from build123d import *

# Parameters (mm, degrees)
SKETCH1_W           = 76
SKETCH1_H           = 13
SKETCH1_W_2         = 74.5
SKETCH1_H_2         = 11.5
BOSS_EXTRUDE1_DEPTH = 2.5
SKETCH2_R           = 1.6
CUT_EXTRUDE1_DEPTH  = 41.239905566
BOSS_EXTRUDE2_REACH = 42.004
SKETCH3_R           = 1


with BuildPart() as part:
    # Sketch1 → Boss-Extrude1 (new, symmetric)
    with BuildSketch(Plane(origin=(0, 0, 0), x_dir=(1, 0, 0), z_dir=(0, 1, 0))):
        Rectangle(SKETCH1_W, SKETCH1_H)
        Rectangle(SKETCH1_W_2, SKETCH1_H_2, mode=Mode.SUBTRACT)
    extrude(amount=BOSS_EXTRUDE1_DEPTH, both=True)

    # Sketch2 → Cut-Extrude1 (cut, through all)
    with BuildSketch(Plane.XY.offset(6.5)):
        with Locations((23, 0)):
            Circle(SKETCH2_R)
        with BuildLine():
            Line((-25, 1.15), (8.6, 1.15))
            ThreePointArc((8.6, 1.15), (9.75, 0), (8.6, -1.15))
            Line((8.6, -1.15), (-25, -1.15))
            ThreePointArc((-25, -1.15), (-26.15, 0), (-25, 1.15))
        make_face()
    extrude(amount=-CUT_EXTRUDE1_DEPTH, mode=Mode.SUBTRACT)

    # Sketch3 → Boss-Extrude2 (add, up to next)
    with BuildSketch(Plane.XY.offset(-5.75), mode=Mode.PRIVATE) as boss_extrude2_sk1:
        with Locations(Location((-31, 0, 0), (0, 0, 180))):
            Circle(SKETCH3_R)
    boss_extrude2_tool1 = extrude(boss_extrude2_sk1.sketch, amount=BOSS_EXTRUDE2_REACH, mode=Mode.PRIVATE) - part.part
    add(boss_extrude2_tool1.solids().sort_by_distance((-31, 0, -5.75))[0])


solid = part.part
Source: CAD feature listing. Evaluate the final solid. Frame: model axes, mm. A direction names the side the tool comes from. Give positions to 0.01 mm unless a question says otherwise; leave off trailing zeros. Loops run counter-clockwise (first coordinate to the right, second up) from the corner with the lowest first, then second, coordinate; pieces in that order, holes last. Notation, with made-up numbers: (-21, -39) -> (-12, -39) arc R20 cw to (-12, -11) -> close; hole circle Ø1 at (23, 16). An arc over 180 degrees is marked (long way). Use a Markdown table: item, result. Add a question column.
1) Reachability of faces 5 (the face through (-37.25, 0, 0)), 6 (the face through (-38, 0, 0)), 7 (the face through (-30, 0, 0)) from +Z, -Z, +X, -X, +Y, -Y: full face, straight path, thin tool, end or side. Return the list, or none.
2) Pull-direction query (Y, two-part tool) for faces 1 (the face through (24.526, 0.481, -6.12)), 2 (the face through (0, -2.5, -6)), 3 (the face through (-1, -2, -6.5)), 4 (the face through (24.526, 0.481, 6.13)); classes: +Y half, -Y half, draft (parallel to the pull), parting line (faces both ways), or undercut.
3) Section query A-A, the plane y = 0. Return the cut outline in (x, z), then the cut area to 3 significant figures.
4) Line query: line 1 along X through (y, z) = (-0.15, -5.5); line 2 along Y through (x, z) = (23, -6.2); line 3 along Z through (x, y) = (11.5, 0.45). Output: solid intervals per line, ascending. Write a range as [from, to].
5) Section query C-C, the plane z = -3.25. Return the cut outline in (x, y).
6) Section query B-B, the plane x = 23. Return the cut outline in (y, z), then the cut area to 3 significant figures.
Numbers:
| question | item | result |
|---|---|---|
| 1 | face 5 | +Y, -Y |
| 1 | face 6 | +Z, -Z, -X, +Y, -Y |
| 1 | face 7 | none |
| 2 | face 1 | undercut |
| 2 | face 2 | -Y half |
| 2 | face 3 | draft |
| 2 | face 4 | undercut |
| 3 | outline | (-38, -6.5) -> (-26.15, -6.5) -> (-26.15, -5.75) -> (-30, -5.75) -> (-30, 5.75) -> (-26.15, 5.75) -> (-26.15, 6.5) -> (-38, 6.5) -> close; (9.75, -6.5) -> (21.4, -6.5) -> (21.4, -5.75) -> (9.75, -5.75) -> close; (9.75, 5.75) -> (21.4, 5.75) -> (21.4, 6.5) -> (9.75, 6.5) -> close; (24.6, -6.5) -> (38, -6.5) -> (38, 6.5) -> (24.6, 6.5) -> (24.6, 5.75) -> (37.25, 5.75) -> (37.25, -5.75) -> (24.6, -5.75) -> close; hole (-37.25, -5.75) -> (-32, -5.75) -> (-32, 5.75) -> (-37.25, 5.75) -> close |
| 3 | area | 95.6 mm2 |
| 4 | line 1 | x = [-38, -37.25], [-31.99, -30.01], [37.25, 38] |
| 4 | line 2 | y = [-2.5, -1.6], [1.6, 2.5] |
| 4 | line 3 | z = [-6.5, -5.75], [5.75, 6.5] |
| 5 | outline | (-38, -2.5) -> (-37.25, -2.5) -> (-37.25, 2.5) -> (-38, 2.5) -> close; circle Ø2 at (-31, 0); (37.25, -2.5) -> (38, -2.5) -> (38, 2.5) -> (37.25, 2.5) -> close |
| 6 | outline | (-2.5, -6.5) -> (-1.6, -6.5) -> (-1.6, -5.75) -> (-2.5, -5.75) -> close; (-2.5, 5.75) -> (-1.6, 5.75) -> (-1.6, 6.5) -> (-2.5, 6.5) -> close; (1.6, -6.5) -> (2.5, -6.5) -> (2.5, -5.75) -> (1.6, -5.75) -> close; (1.6, 5.75) -> (2.5, 5.75) -> (2.5, 6.5) -> (1.6, 6.5) -> close |
| 6 | area | 2.70 mm2 |
